from build123d import *

# Parameters (mm, degrees)
CROQUIS1_R              = 3
SALIENTE_EXTRUIR1_DEPTH = 27.1
CORTAR_EXTRUIR1_DEPTH   = 12
CHAFL_N1_SIZE           = 0.25
CUT_EXTRUDE2_DEPTH      = 2.5
CHAMFER1_SIZE           = 0.5
FILLET1_R               = 0.25


with BuildPart() as part:
    # Croquis1 → Saliente-Extruir1 (new body)
    with BuildSketch(Plane.XY):
        Circle(CROQUIS1_R)
    extrude(amount=SALIENTE_EXTRUIR1_DEPTH)

    # Croquis2 → Cortar-Extruir1 (cut)
    with BuildSketch(Plane.XY.offset(27.1)):
        with BuildLine():
            Line((-1.8, 2.4), (1.8, 2.4))
            ThreePointArc((1.8, 2.4), (0, 3), (-1.8, 2.4))
        make_face()
    extrude(amount=-CORTAR_EXTRUIR1_DEPTH, mode=Mode.SUBTRACT)

    # Chaflán1
    chafl_n1_edges = [part.edges().sort_by_distance(p)[0] for p in [
        (-1.341640786, -2.683281573, 27.1),
    ]]
    chamfer(chafl_n1_edges, length=CHAFL_N1_SIZE)

    # Sketch1 → Cut-Extrude2 (cut)
    with BuildSketch(Plane(origin=(0, 0, 0), x_dir=(-1, 0, 0), z_dir=(0, 0, -1))):
        with BuildLine():
            Line((0, 0.75), (-0.661437828, 0.75))
            ThreePointArc((-0.661437828, 0.75), (0, -1), (0.661437828, 0.75))
            Line((0.661437828, 0.75), (0, 0.75))
        make_face()
    extrude(amount=-CUT_EXTRUDE2_DEPTH, mode=Mode.SUBTRACT)

    # Chamfer1
    chamfer1_edges = [part.edges().sort_by_distance(p)[0] for p in [
        (-3, 0, 0),
    ]]
    chamfer(chamfer1_edges, length=CHAMFER1_SIZE)

    # Fillet1
    fillet1_edges = [part.edges().sort_by_distance(p)[0] for p in [
        (0, 2.4, 15.1),
    ]]
    fillet(fillet1_edges, radius=FILLET1_R)


solid = part.part
Model file for the job. Use its own axes, mm. A direction names the side the tool comes from. Round coordinates to 2 decimals unless told otherwise and drop trailing zeros. Order: outer loops, then holes, each group sorted by start corner. A loop starts at its lowest first (then second) coordinate and runs counter-clockwise, first axis right, second up. Notation, with made-up numbers: M 46,-25 L 59,-25 A35 cw 59,12 Z; hole C 33.25,-15.75 d7. An arc over 180 degrees is marked long. Write each question's results on one line, items separated by ' | '. Start each with the question number.
(1) Saw through at B-B, the plane x = 0. Give the cut face in (y, z).
(2) Which spindle directions (+Z, -Z, +X, -X, +Y, -Y) get a long thin tool onto all of the face, cutting with end or side? Do faces 1 (the face through (0, -1, 1)), 2 (the face through (-0.11, -2.87, 26.98)), 3 (the face through (0, 2.4, 21)). Say none if no direction does.
(3) Drop flat-ended pins along their axis: pin 1 (1.5 mm diameter, centred on y = -2, z = 11.5, fed in from +X); pin 2 (3 mm diameter, centred on x = 0.5, z = 21, fed in from +Y). Give the stop position or say it passes through.
(4) Probe probe 1 along X at (y, z) = (0, 0.8); probe 2 along Z at (x, y) = (0.5, -0.75); probe 3 along Z at (x, y) = (-1.5, -2.25). List the from-to ranges inside material, lowest first. Write a range as from..to.
(5) Saw through at A-A, the plane y = 0. Give the cut face in (x, z).
(6) Saw through at C-C, the plane z = 9. Give the cut face in (x, y).
(7) Two-plate mould, pull along Y, no slides. Class faces 4 (the face through (-0.65, -2.93, 13.49)), 5 (the face through (0, 0, 2.5)), 6 (the face through (0, 0, 27.1)): pulls with the +Y half, pulls with the -Y half, needs draft (parallel to the pull), parting line crosses it, or undercut.
Established:
1) outline: M -3,0.5 L -2.5,0 L -1,0 L -1,2.5 L 0.75,2.5 L 0.75,0 L 2.5,0 L 3,0.5 L 3,15.1 L 2.65,15.1 A0.25 cw 2.4,15.35 L 2.4,27.1 L -2.75,27.1 L -3,26.85 Z
2) face 1: -Z | face 2: +Z | face 3: +Z, +X, -X, +Y
3) pin 1: stops at x = 2.73 | pin 2: stops at y = 2.4
4) probe 1: x = -3..-1, 1..3 | probe 2: z = 2.5..27.1 | probe 3: z = 0.2..27.1
5) outline: M -3,0.5 L -2.5,0 L -1,0 L -1,2.5 L 1,2.5 L 1,0 L 2.5,0 L 3,0.5 L 3,26.85 L 2.75,27.1 L -2.75,27.1 L -3,26.85 Z
6) outline: C 0,0 d6
7) face 4: parting line crosses it | face 5: undercut | face 6: needs draft
